```python
from build123d import *

# Parameters (mm, degrees)
F0_W     = 76.962
F0_H     = 28.321
F0_W_2   = 45.72
F0_W_3   = 25.4
F0_H_2   = 25.4
F1_DEPTH = 53.721
F3_DEPTH = 25.4
F4_DEPTH = 53.721
F5_R     = 6.985
F6_DEPTH = 25.4
F7_DEPTH = 28.321


with BuildPart() as f1:
    # F0 (on Top) → F1 (new body)
    with BuildSketch(Plane.XY):
        Polygon((86.741, -28.321), (61.341, -28.321), (-15.621, -28.321), (-61.341, -28.321), (-61.341, 0), (-61.341, 28.321), (-15.621, 28.321), (61.341, 28.321), (86.741, 28.321), (86.741, 53.721), (-86.741, 53.721), (-86.741, -53.721), (86.741, -53.721), align=None)
        with Locations((22.86, -14.1605)):
            Rectangle(F0_W, F0_H)
        with Locations((-38.481, -14.1605)):
            Rectangle(F0_W_2, F0_H)
        with Locations((74.041, -14.1605)):
            Rectangle(F0_W_3, F0_H)
        with Locations((74.041, 14.1605)):
            Rectangle(F0_W_3, F0_H)
        with Locations((22.86, 14.1605)):
            Rectangle(F0_W, F0_H)
        with Locations((-38.481, 14.1605)):
            Rectangle(F0_W_2, F0_H)
        Polygon((112.141, 0), (112.141, -28.321), (112.141, -53.721), (137.541, -53.721), (137.541, 53.721), (112.141, 53.721), (112.141, 28.321), align=None)
        with Locations((99.441, 41.021)):
            Rectangle(F0_W_3, F0_H_2)
        with Locations((99.441, -41.021)):
            Rectangle(F0_W_3, F0_H_2)
        with Locations((99.441, -14.1605)):
            Rectangle(F0_W_3, F0_H)
        with Locations((99.441, 14.1605)):
            Rectangle(F0_W_3, F0_H)
    extrude(amount=-F1_DEPTH)

    # F0 (on Top) → F2 (revolve, cut)
    with BuildSketch(Plane.XY):
        with Locations((74.041, 14.1605)):
            Rectangle(F0_W_3, F0_H)
        with Locations((-38.481, 14.1605)):
            Rectangle(F0_W_2, F0_H)
        with Locations((22.86, 14.1605)):
            Rectangle(F0_W, F0_H)
    revolve(axis=Axis((0, 0, 0), (1, 0, 0)), mode=Mode.SUBTRACT)

    # F0 (on Top) → F3 (join)
    with BuildSketch(Plane.XY):
        Polygon((86.741, -28.321), (61.341, -28.321), (-15.621, -28.321), (-61.341, -28.321), (-61.341, 0), (-61.341, 28.321), (-15.621, 28.321), (61.341, 28.321), (86.741, 28.321), (86.741, 53.721), (-86.741, 53.721), (-86.741, -53.721), (86.741, -53.721), align=None)
        Polygon((112.141, 0), (112.141, -28.321), (112.141, -53.721), (137.541, -53.721), (137.541, 53.721), (112.141, 53.721), (112.141, 28.321), align=None)
    extrude(amount=F3_DEPTH)

    # F0 (on Top) → F4 (cut)
    with BuildSketch(Plane.XY):
        with Locations((-38.481, 14.1605)):
            Rectangle(F0_W_2, F0_H)
        with Locations((-38.481, -14.1605)):
            Rectangle(F0_W_2, F0_H)
    extrude(amount=-F4_DEPTH, mode=Mode.SUBTRACT)

    # F5 (on face) → F6 (cut)
    with BuildSketch(Plane.YZ.offset(137.541)):
        Circle(F5_R)
    extrude(amount=-F6_DEPTH, mode=Mode.SUBTRACT)

    # F0 (on Top) → F7 (cut)
    with BuildSketch(Plane.XY):
        with Locations((99.441, 41.021)):
            Rectangle(F0_W_3, F0_H_2)
        with Locations((99.441, 14.1605)):
            Rectangle(F0_W_3, F0_H)
        with Locations((99.441, -14.1605)):
            Rectangle(F0_W_3, F0_H)
        with Locations((99.441, -41.021)):
            Rectangle(F0_W_3, F0_H_2)
    extrude(amount=-F7_DEPTH, mode=Mode.SUBTRACT)


solid = f1.part
```
Work out the finished part from the listing and answer in its coordinate system (mm). A direction names the side the tool comes from. Give positions to 0.01 mm unless a question says otherwise; leave off trailing zeros. Write each loop counter-clockwise with the first axis right and the second up, starting at its lowest first coordinate (ties: lowest second). Pieces come first, ordered by that corner, then holes. Notation, with made-up numbers: (-21.75, 51) - (25.25, 51) arc R25 cw to (25.25, 88) - close; hole circle Ø1 at (42.5, -9.5). An arc over 180 degrees is marked (long way). Use one line per item in the form item = value.
1. A cutting plane is placed at C-C (y = 11). Write down the section's boundary in (x, z).
Filled in:
outline = (-86.74, -53.72) - (-61.34, -53.72) - (-61.34, 25.4) - (-86.74, 25.4) - close; (-15.62, -53.72) - (137.54, -53.72) - (137.54, 25.4) - (112.14, 25.4) - (112.14, -28.32) - (86.74, -28.32) - (86.74, -26.1) - (-15.62, -26.1) - close
2. A cutting plane is placed at B-B (z = 18). Write down the section's boundary in (x, y), and give its area (3 significant figures).
Filled in:
outline = (-86.74, -53.72) - (86.74, -53.72) - (86.74, -28.32) - (-61.34, -28.32) - (-61.34, 28.32) - (86.74, 28.32) - (86.74, 53.72) - (-86.74, 53.72) - close; (112.14, -53.72) - (137.54, -53.72) - (137.54, 53.72) - (112.14, 53.72) - close
area = 13,000 mm^2
3. A cutting plane is placed at A-A (x = -26.5). Write down the section's boundary in (y, z), and give its area (3 significant figures).
Filled in:
outline = (-53.72, -53.72) - (-28.32, -53.72) - (-28.32, 25.4) - (-53.72, 25.4) - close; (28.32, -53.72) - (53.72, -53.72) - (53.72, 25.4) - (28.32, 25.4) - close
area = 4,020 mm^2
4. Consider L1, parallel to X at y = -23, z = -22; L2, parallel to X at y = 8.5, z = -4; L3, parallel to Y at x = 59.5, z = 22. Determine where each line is inside the solid, lowest interval first.
Filled in:
L1 = -86.74 to -61.34, -15.62 to 86.74, 112.14 to 137.54
L2 = -86.74 to -61.34, 112.14 to 137.54
L3 = -53.72 to -28.32, 28.32 to 53.72
5. Determine the mould class of faces 1 (the face through (-3, -28.321, 3)), 2 (the face through (137.541, -1, -14)), 3 (the face through (24, -53.721, -15)) for opening direction Y: released by +Y, released by -Y, zero draft, split by the parting line, or undercut.
Filled in:
face_1 = undercut
face_2 = zero draft
face_3 = released by -Y
6. A cutting plane is placed at D-D (x = 123.5). Write down the section's boundary in (y, z) (3 decimals), and give its area (3 significant figures).
Filled in:
outline = (-53.721, -53.721) - (53.721, -53.721) - (53.721, 25.4) - (-53.721, 25.4) - close; hole circle Ø13.97 at (0, 0)
area = 8,350 mm^2
7. For faces 4 (the face through (125.019, -0.909, 6.926)), 5 (the face through (86.741, 38, -2)), 6 (the face through (34.843, -0.623, -28.314)), 7 (the face through (-61.341, 0, -15)), 8 (the face through (125, 1, 25.4)), determine the directions among +Z, -Z, +X, -X, +Y, -Y from which every point of the face is accessible in a straight line to the end or side of a thin tool.
Filled in:
face_4 = +X
face_5 = +Z, +Y, -Y
face_6 = +Z
face_7 = +Z, -Z
face_8 = +Z, +X, -X, +Y, -Y
